CAD build for the part. Positions are in the model's coordinates, mm. A direction names the side the tool comes from. Round coordinates to 2 decimals unless told otherwise and drop trailing zeros. Write each loop counter-clockwise with the first axis right and the second up, starting at its lowest first coordinate (ties: lowest second). Pieces come first, ordered by that corner, then holes. Notation, with made-up numbers: (-22, 24) -> (-1, 24) arc R34 cw to (-1, 59) -> close; hole circle Ø7 at (30, 81.25). An arc over 180 degrees is marked (long way). Put each result on its own line as item: value. Start each with the question number.
1. Saw through at C-C on z = 69.5. List the corners of the cut face in (x, y).
2. Pull direction Z, two halves, no side cores. Call faces 1 (the cylindrical face through (4.53, 6.65, 86.36)), 2 (the flat face through (7, 23.5, 69)), 3 (the flat face through (9, 18, 0)): pulls with the +Z half, pulls with the -Z half, needs draft (parallel to the pull), parting line crosses it, or undercut.
3. Flat gauge pins, fed straight in: P1, Ø4, axis at x = 6.58, y = 18, coming from the +Z side; P2, Ø4, axis at x = 8.5, z = 71, coming from the +Y side; P3, Ø3.5, axis at x = 6.58, y = 18, coming from the +Z side. Where does each tip first touch, or does it go through?
4. Saw through at A-A on y = 30. List the corners of the cut face in (x, z) (3 decimals), and give its area (3 significant figures).
5. Drill centre lines: line 1 (X direction, y = 30, z = 82) (3 decimals); line 2 (Z direction, x = 5, y = 33); line 3 (Y direction, x = 7, z = 9). Where is each one in solid material? Low to high. Write a range as from..to.
6. 3-axis set-ups, long thin cutter, end or side, ignore diameter. For faces 4 (the cylindrical face through (4.99, 7.45, 2.54)), 5 (the cylindrical face through (0.86, 34.1, 83.48)), 6 (the cylindrical face through (5.59, 16.09, 86.36)), 7 (the flat face through (5, 27, 77.9)): which of +Z, -Z, +X, -X, +Y, -Y reach the whole face in a straight line?
7. Saw through at B-B on z = 54. List the corners of the cut face in (x, y) (3 decimals).
from build123d import *

# Parameters (mm, degrees)
SKETCH1_W                = 13
SKETCH1_H                = 35
SKETCH1_R                = 3.175
BOSS_EXTRUDE1_DEPTH      = 88.9
CUT_EXTRUDE1_DEPTH       = 9
M4_CLEARANCE_HOLE1_D     = 4.3
M4_CLEARANCE_HOLE1_DEPTH = 5
M4_CLEARANCE_HOLE1_TIP   = 1.291850331
M4_CLEARANCE_HOLE2_D     = 4.3
M4_CLEARANCE_HOLE2_DEPTH = 5
M4_CLEARANCE_HOLE2_TIP   = 1.291850331
FILLET1_R                = 3


with BuildPart() as part:
    # Sketch1 → Boss-Extrude1 (new body)
    with BuildSketch(Plane.XY):
        with Locations((6.5, 17.5)):
            Rectangle(SKETCH1_W, SKETCH1_H)
        with Locations((6.5, 30)):
            Circle(SKETCH1_R, mode=Mode.SUBTRACT)
    extrude(amount=BOSS_EXTRUDE1_DEPTH)

    # Sketch2 → Cut-Extrude1 (cut, symmetric)
    with BuildSketch(Plane.XY.offset(68.9)):
        Polygon((0, 30), (0, 35), (13, 35), (13, 30), (13, 23.5), (0, 23.5), align=None)
    extrude(amount=CUT_EXTRUDE1_DEPTH, both=True, mode=Mode.SUBTRACT)

    # M4 Clearance Hole1
    with Locations(Plane(origin=(0, 0, 0), x_dir=(-1, 0, 0), z_dir=(0, 0, -1))):
        with Locations((-6.579246302, 18), (-6.579246302, 6)):
            Hole(M4_CLEARANCE_HOLE1_D / 2, depth=M4_CLEARANCE_HOLE1_DEPTH)
            with Locations((0, 0, -(M4_CLEARANCE_HOLE1_DEPTH + M4_CLEARANCE_HOLE1_TIP / 2))):  # 118° drill point
                Cone(0, M4_CLEARANCE_HOLE1_D / 2, M4_CLEARANCE_HOLE1_TIP, mode=Mode.SUBTRACT)

    # M4 Clearance Hole2
    with Locations(Plane.XY.offset(88.9)):
        with Locations((6.579246302, 18), (6.579246302, 6)):
            Hole(M4_CLEARANCE_HOLE2_D / 2, depth=M4_CLEARANCE_HOLE2_DEPTH)
            with Locations((0, 0, -(M4_CLEARANCE_HOLE2_DEPTH + M4_CLEARANCE_HOLE2_TIP / 2))):  # 118° drill point
                Cone(0, M4_CLEARANCE_HOLE2_D / 2, M4_CLEARANCE_HOLE2_TIP, mode=Mode.SUBTRACT)

    # Fillet1
    fillet1_edges = [part.edges().sort_by_distance(p)[0] for p in [
        (0, 35, 29.95),
        (13, 35, 29.95),
        (0, 35, 83.4),
        (13, 35, 83.4),
        (13, 0, 44.45),
        (0, 0, 44.45),
    ]]
    fillet(fillet1_edges, radius=FILLET1_R)


solid = part.part
Return value:
1. outline: (0, 3) arc R3 ccw to (3, 0) -> (10, 0) arc R3 ccw to (13, 3) -> (13, 23.5) -> (0, 23.5) -> close
2. face 1: needs draft
2. face 2: undercut
2. face 3: pulls with the -Z half
3. P1: stops at z = 83.81
3. P2: stops at y = 23.5
3. P3: stops at z = 83.66
4. outline: (0, 0) -> (3.325, 0) -> (3.325, 59.9) -> (0, 59.9) -> close; (0, 77.9) -> (3.325, 77.9) -> (3.325, 88.9) -> (0, 88.9) -> close; (9.675, 0) -> (13, 0) -> (13, 59.9) -> (9.675, 59.9) -> close; (9.675, 77.9) -> (13, 77.9) -> (13, 88.9) -> (9.675, 88.9) -> close
4. area: 471 mm^2
5. line 1: x = 0..3.325, 9.675..13
5. line 2: z = 0..59.9, 77.9..88.9
5. line 3: y = 0..26.86, 33.14..35
6. face 4: -Z
6. face 5: +Z, -Z, -X, +Y
6. face 6: +Z
6. face 7: +X, -X, +Y
7. outline: (0, 3) arc R3 ccw to (3, 0) -> (10, 0) arc R3 ccw to (13, 3) -> (13, 32) arc R3 ccw to (10, 35) -> (3, 35) arc R3 ccw to (0, 32) -> close; hole circle Ø6.35 at (6.5, 30)
